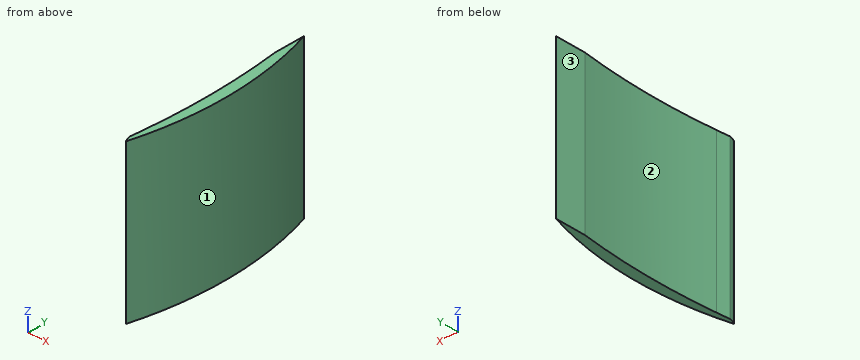
from build123d import *

# Parameters (mm, degrees)
F0_W     = 5
F0_H     = 54
F1_DEPTH = 40
F3_DEPTH = 40
F4_DEPTH = 40
F5_DEPTH = 40


with BuildPart() as f1:
    # F0 (on Top) → F1 (new body)
    with BuildSketch(Plane.XY):
        Rectangle(F0_W, F0_H)
    extrude(amount=F1_DEPTH)

    # F2 (on face) → F3 (cut)
    with BuildSketch(Plane.XY.offset(40)):
        with BuildLine():
            ThreePointArc((-1.750376, -18.09707), (-1.121, 0.471757), (-2.5, 19))
            Line((-2.5, 19), (-2.5, -25))
            ThreePointArc((-2.5, -25), (-2.281968, -23.239421), (-2.082123, -21.476685))
            ThreePointArc((-2.082123, -21.476685), (-2.160412, -19.76291), (-1.750376, -18.09707))
        make_face()
    extrude(amount=-F3_DEPTH, mode=Mode.SUBTRACT)

    # F2 (on face) → F4 (join)
    with BuildSketch(Plane.XY.offset(40)):
        with BuildLine():
            ThreePointArc((-1.415606, -23.295218), (1.646941, 1.930112), (-2.5, 27))
            Line((-2.5, 27), (-2.5, 19))
            ThreePointArc((-2.5, 19), (-1.121, 0.471757), (-1.750376, -18.09707))
            ThreePointArc((-1.750376, -18.09707), (-1.907901, -19.787697), (-2.082123, -21.476685))
            ThreePointArc((-2.082123, -21.476685), (-1.82275, -22.413031), (-1.415606, -23.295218))
        make_face()
    extrude(amount=F4_DEPTH)

    # F1_face (on face) → F5 (cut)
    with BuildSketch(Plane.XY.offset(40)):
        with BuildLine():
            Line((2.5, 27), (2.5, -27))
            Line((2.5, -27), (-2.5, -27))
            Line((-2.5, -27), (-2.5, -25))
            ThreePointArc((-2.5, -25), (-2.281968, -23.239421), (-2.082123, -21.476685))
            ThreePointArc((-2.082123, -21.476685), (-2.160412, -19.76291), (-1.750376, -18.09707))
            ThreePointArc((-1.750376, -18.09707), (-1.121, 0.471757), (-2.5, 19))
            Line((-2.5, 19), (-2.5, 27))
            Line((-2.5, 27), (2.5, 27))
        make_face()
    extrude(amount=-F5_DEPTH, mode=Mode.SUBTRACT)


solid = f1.part
CAD build for the part. Positions are in the model's coordinates, mm. Face numbers are marked on the shaded views. Give positions to 0.01 mm unless a question says otherwise; leave off trailing zeros. Order: outer loops, then holes, each group sorted by start corner. A loop starts at its lowest first (then second) coordinate and runs counter-clockwise, first axis right, second up. Notation, with made-up numbers: (87, -0.5) - (101, -0.5) arc R25 ccw to (101, 22.5) - close; hole circle Ø6 at (73, 65.5). An arc over 180 degrees is marked (long way). Answer in a Markdown table with one row per item.
1. Saw through at C-C, the plane y = 15.5. Give the cut face in (x, z), plus the area to 3 significant figures.
Data:
| item | result |
|---|---|
| outline | (-2.08, 40) - (0.32, 40) - (0.32, 80) - (-2.08, 80) - close |
| area | 96.0 mm² |
2. Pull direction Y, two halves, no side cores. Call the marked faces 1, 2 and 3: pulls with the +Y half, pulls with the -Y half, needs draft (parallel to the pull), parting line crosses it, or undercut.
Data:
| item | result |
|---|---|
| face 1 | parting line crosses it |
| face 2 | undercut |
| face 3 | needs draft |
3. Probe probe 1 along X at (y, z) = (21, 50); probe 2 along X at (y, z) = (15.5, 63). List the from-to ranges inside material, lowest first. Write a range as [from, to].
Data:
| item | result |
|---|---|
| probe 1 | x = [-2.5, -0.83] |
| probe 2 | x = [-2.08, 0.32] |
4. Flat gauge pins, fed straight in: pin 1 (8 mm diameter, centred on y = 9, z = 47, fed in from -X); pin 2 (2 mm diameter, centred on y = 20, z = 69.5, fed in from +X); pin 3 (5 mm diameter, centred on y = -10.5, z = 48.5, fed in from +X). Where does each tip first touch, or does it go through?
Data:
| item | result |
|---|---|
| pin 1 | stops at x = -1.83 |
| pin 2 | stops at x = -0.37 |
| pin 3 | stops at x = 1.31 |
5. Saw through at A-A, the plane z = 55.5. Give the cut face in (x, y).
Data:
| item | result |
|---|---|
| outline | (-2.5, 19) arc R171.84 cw to (-1.75, -18.1) arc R171.84 cw to (-2.08, -21.48) arc R6 ccw to (-1.42, -23.3) arc R89.54 ccw to (-2.5, 27) - close |
